from build123d import *

# Parameters (mm, degrees)
BOSS_EXTRUDE1_DEPTH = 6
SKETCH2_W           = 20
SKETCH2_H           = 20
SKETCH2_R           = 5
BOSS_EXTRUDE2_DEPTH = 20


with BuildPart() as part:
    # Sketch1 → Boss-Extrude1 (new body)
    with BuildSketch(Plane(origin=(0, 0, 0), x_dir=(1, 0, 0), z_dir=(0, 1, 0))):
        Polygon((-34.039277024, -34.17435352), (115.960722976, -34.17435352), (115.960722976, 85.82564648), (40.960722976, 160.82564648), (-34.039277024, 85.82564648), align=None)
    extrude(amount=BOSS_EXTRUDE1_DEPTH)

    # Sketch2 → Boss-Extrude2 (add)
    with BuildSketch(Plane(origin=(0, 6, 0), x_dir=(1, 0, 0), z_dir=(0, 1, 0))):
        with Locations((40.960722976, -24.206365995)):
            Rectangle(SKETCH2_W, SKETCH2_H)
        with Locations(Location((40.960722976, -24.206365995, 0), (0, 0, 270))):
            Circle(SKETCH2_R, mode=Mode.SUBTRACT)
    extrude(amount=BOSS_EXTRUDE2_DEPTH)


solid = part.part
Geometry check sheet. Reference: the model listing, model coordinates, mm. A direction names the side the tool comes from. Give positions to 0.01 mm unless a question says otherwise; leave off trailing zeros. Write each loop counter-clockwise with the first axis right and the second up, starting at its lowest first coordinate (ties: lowest second). Pieces come first, ordered by that corner, then holes.
1) Set-up check for faces 1 (the face through (78.986, 2.958, -122.801)), 2 (the face through (50.961, 16, 24)), 3 (the face through (41, 6, 24)), 4 (the face through (41, 16, 14.206)), 5 (the face through (30.961, 16, 24)): record each of +Z, -Z, +X, -X, +Y, -Y from which the full face is reachable in a straight line by a thin tool's end or side.
Values follow:
face 1: -Z, +X, +Y, -Y
face 2: +Z, -Z, +X, +Y
face 3: +Y
face 4: -Z, +X, -X, +Y
face 5: +Z, -Z, -X, +Y
2) Thickness scan on line 1 (Y direction, x = 56, z = 16.5); line 2 (Z direction, x = 32, y = 21.5); line 3 (X direction, y = 16.75, z = 21). Record the ranges inside material, lowest first.
Values follow:
line 1: y = 0 to 6
line 2: z = 14.21 to 34.21
line 3: x = 30.96 to 37.12, 44.8 to 50.96
3) Cross-section at B-B (y = 12.75). Record the boundary of the cut face in (x, z).
Values follow:
outline: (30.96, 14.21) - (50.96, 14.21) - (50.96, 34.21) - (30.96, 34.21) - close; hole circle Ø10 at (40.96, 24.21)
4) Cross-section at A-A (z = 16.5). Record the boundary of the cut face in (x, y), plus the area to 3 significant figures.
Values follow:
outline: (-34.04, 0) - (115.96, 0) - (115.96, 6) - (50.96, 6) - (50.96, 26) - (30.96, 26) - (30.96, 6) - (-34.04, 6) - close
area: 1,300 mm2
5) Go/stop test with flat-tipped pins: pin 1 Ø3 at (x, z) = (40, 26) entering from +Y; pin 2 Ø1.8 at (x, y) = (12.5, 4) entering from +Z; pin 3 Ø8 at (x, y) = (80, 9.5) entering from -Z. Record where each tip stops, or that it passes through.
Values follow:
pin 1: stops at y = 6
pin 2: stops at z = 34.17
pin 3: stops at z = -123.72
6) Cross-section at C-C (y = 2.25). Record the boundary of the cut face in (x, z), plus the area to 3 significant figures.
Values follow:
outline: (-34.04, -85.83) - (40.96, -160.83) - (115.96, -85.83) - (115.96, 34.17) - (-34.04, 34.17) - close
area: 23,600 mm2
7) Release check for a two-part mould opening along Z. For faces 6 (the face through (45.18, 15.86, 26.89)), 7 (the face through (40, 3, 34.174)), 8 (the face through (40, 6, -43)) record: released by +Z, released by -Z, zero draft, split by the parting line, or undercut.
Values follow:
face 6: undercut
face 7: released by +Z
face 8: zero draft
